```python
from build123d import *

# Parameters (mm, degrees)
SKETCH1_W               = 14
SKETCH1_H               = 15
BOSS_EXTRUDE1_DEPTH     = 4
SKETCH2_R               = 3
SKETCH2_R_2             = 1.5
CUT_EXTRUDE1_DEPTH      = 1
CUT_EXTRUDE1_DEPTH_BACK = 5
FILLET1_R               = 2
CUT_EXTRUDE2_START      = -0.2
SKETCH3_W               = 4
SKETCH3_H               = 6
CUT_EXTRUDE2_DEPTH      = 1.2
LPATTERN1_COUNT         = 4
LPATTERN1_PITCH         = 6.666666667
MIRROR1_START           = -0.2
MIRROR1_COPY_1_SKETCH_W = 4
MIRROR1_COPY_1_SKETCH_H = 6
MIRROR1_COPY_1_DEPTH    = 1.2
MIRROR1_COPY_2_SKETCH_W = 4
MIRROR1_COPY_2_SKETCH_H = 6
MIRROR1_COPY_2_DEPTH    = 1.2
MIRROR1_COPY_3_SKETCH_W = 4
MIRROR1_COPY_3_SKETCH_H = 6
MIRROR1_COPY_3_DEPTH    = 1.2
SKETCH4_W               = 6
SKETCH4_H               = 4
CUT_EXTRUDE3_DEPTH      = 1
CUT_EXTRUDE3_DEPTH_BACK = 0.2


with BuildPart() as part:
    # Sketch1 → Boss-Extrude1 (new body)
    with BuildSketch(Plane(origin=(0, 0, 0), x_dir=(1, 0, 0), z_dir=(0, 1, 0))):
        Polygon((-11, 18), (-11, 7.5), (-11, -7.5), (-11, -18), (25, -18), (25, 18), align=None)
        with Locations((-18, 0)):
            Rectangle(SKETCH1_W, SKETCH1_H)
    extrude(amount=BOSS_EXTRUDE1_DEPTH)

    # Sketch2 → Cut-Extrude1 (cut, two sides)
    with BuildSketch(Plane(origin=(0, 4, 0), x_dir=(1, 0, 0), z_dir=(0, 1, 0))) as cut_extrude1_sk:
        with Locations((-18, 3.75)):
            Circle(SKETCH2_R)
        with Locations((-8.25, 15.25)):
            Circle(SKETCH2_R_2)
        with Locations((22.25, 15.25)):
            Circle(SKETCH2_R_2)
        with Locations((-18, -3.75)):
            Circle(SKETCH2_R)
        with Locations((22.25, -15.25)):
            Circle(SKETCH2_R_2)
        with Locations((-8.25, -15.25)):
            Circle(SKETCH2_R_2)
    extrude(amount=CUT_EXTRUDE1_DEPTH, mode=Mode.SUBTRACT)
    extrude(cut_extrude1_sk.sketch, amount=-CUT_EXTRUDE1_DEPTH_BACK, mode=Mode.SUBTRACT)

    # Fillet1
    fillet1_edges = [part.edges().sort_by_distance(p)[0] for p in [
        (-11, 2, -18),
        (25, 2, -18),
        (25, 2, 18),
        (-11, 2, 18),
        (-11, 2, 7.5),
        (-25, 2, 7.5),
        (-25, 2, -7.5),
        (-11, 2, -7.5),
    ]]
    fillet(fillet1_edges, radius=FILLET1_R)

    # Sketch3 → Cut-Extrude2 (cut)
    with BuildSketch(Plane(origin=(0, 4, 0), x_dir=(1, 0, 0), z_dir=(0, 1, 0)).offset(CUT_EXTRUDE2_START)):
        with Locations((-3.25, 14)):
            Rectangle(SKETCH3_W, SKETCH3_H)
    cut_extrude2 = extrude(amount=CUT_EXTRUDE2_DEPTH, mode=Mode.SUBTRACT)

    # LPattern1: Cut-Extrude2 ×4
    with Locations(*[(i * LPATTERN1_PITCH, 0, 0) for i in range(1, LPATTERN1_COUNT)]):
        add(cut_extrude2, mode=Mode.SUBTRACT)

    # Mirror1: Cut-Extrude2 across plane
    add(cut_extrude2.mirror(Plane.XY), mode=Mode.SUBTRACT)

    # Mirror1 copy 1 sketch → Mirror1 copy 1 (cut)
    with BuildSketch(Plane(origin=(6.666666667, 4, 0), x_dir=(1, 0, 0), z_dir=(0, 1, 0)).offset(MIRROR1_START)):
        with Locations((-3.25, -14)):
            Rectangle(MIRROR1_COPY_1_SKETCH_W, MIRROR1_COPY_1_SKETCH_H)
    extrude(amount=MIRROR1_COPY_1_DEPTH, mode=Mode.SUBTRACT)

    # Mirror1 copy 2 sketch → Mirror1 copy 2 (cut)
    with BuildSketch(Plane(origin=(13.333333333, 4, 0), x_dir=(1, 0, 0), z_dir=(0, 1, 0)).offset(MIRROR1_START)):
        with Locations((-3.25, -14)):
            Rectangle(MIRROR1_COPY_2_SKETCH_W, MIRROR1_COPY_2_SKETCH_H)
    extrude(amount=MIRROR1_COPY_2_DEPTH, mode=Mode.SUBTRACT)

    # Mirror1 copy 3 sketch → Mirror1 copy 3 (cut)
    with BuildSketch(Plane(origin=(20, 4, 0), x_dir=(1, 0, 0), z_dir=(0, 1, 0)).offset(MIRROR1_START)):
        with Locations((-3.25, -14)):
            Rectangle(MIRROR1_COPY_3_SKETCH_W, MIRROR1_COPY_3_SKETCH_H)
    extrude(amount=MIRROR1_COPY_3_DEPTH, mode=Mode.SUBTRACT)

    # Sketch4 → Cut-Extrude3 (cut, two sides)
    with BuildSketch(Plane(origin=(0, 4, 0), x_dir=(1, 0, 0), z_dir=(0, 1, 0))) as cut_extrude3_sk:
        with Locations((21, 6.5)):
            Rectangle(SKETCH4_W, SKETCH4_H)
        with Locations((-7, 6.5)):
            Rectangle(SKETCH4_W, SKETCH4_H)
        with Locations((-7, -6.5)):
            Rectangle(SKETCH4_W, SKETCH4_H)
        with Locations((21, -6.5)):
            Rectangle(SKETCH4_W, SKETCH4_H)
    extrude(amount=CUT_EXTRUDE3_DEPTH, mode=Mode.SUBTRACT)
    extrude(cut_extrude3_sk.sketch, amount=-CUT_EXTRUDE3_DEPTH_BACK, mode=Mode.SUBTRACT)


solid = part.part
```
For this review, take the finished solid that the model builds, in its own axes (mm). A direction names the side the tool comes from. Round coordinates to 2 decimals unless told otherwise and drop trailing zeros. Write each loop counter-clockwise with the first axis right and the second up, starting at its lowest first coordinate (ties: lowest second). Pieces come first, ordered by that corner, then holes.
1) Mouldability with a two-part tool opening along X and no side actions: class faces 1 (the face through (-3, 3.8, -14)), 2 (the face through (5, 0, 0)), 3 (the face through (-20.997, 2.028, -3.882)), 4 (the face through (25, 2, 0)) as +X half, -X half, draft (parallel to the pull), parting line (faces both ways), or undercut.
Answer below:
face 1: undercut
face 2: draft
face 3: undercut
face 4: +X half
2) Machinability: for faces 5 (the face through (-11.57, 2.03, -8.1)), 6 (the face through (-11, 2, 13)), 7 (the face through (21, 3.8, 6)), which of the approach directions +Z, -Z, +X, -X, +Y, -Y give a long, thin tool a straight path to every point of the face, cutting with its end or side? Answer none if there is none.
Answer below:
face 5: -Z, -X, +Y, -Y
face 6: +Z, -X, +Y, -Y
face 7: +Y
3) Take a section at D-D on z = 15.25. Give the boundary of the cut face in (x, y), then the cut area to 3 significant figures.
Answer below:
outline: (-11, 0) - (-9.75, 0) - (-9.75, 4) - (-11, 4) - close; (-6.75, 0) - (20.75, 0) - (20.75, 4) - (18.75, 4) - (18.75, 3.8) - (14.75, 3.8) - (14.75, 4) - (12.08, 4) - (12.08, 3.8) - (8.08, 3.8) - (8.08, 4) - (5.42, 4) - (5.42, 3.8) - (1.42, 3.8) - (1.42, 4) - (-1.25, 4) - (-1.25, 3.8) - (-5.25, 3.8) - (-5.25, 4) - (-6.75, 4) - close; (23.75, 0) - (25, 0) - (25, 4) - (23.75, 4) - close
area: 117 mm2
4) Take a section at C-C on x = 3.5. Give the boundary of the cut face in (y, z).
Answer below:
outline: (0, -18) - (4, -18) - (4, -17) - (3.8, -17) - (3.8, -11) - (4, -11) - (4, 11) - (3.8, 11) - (3.8, 17) - (4, 17) - (4, 18) - (0, 18) - close
5) Take a section at B-B on z = -3.75. Give the boundary of the cut face in (x, y).
Answer below:
outline: (-25, 0) - (-21, 0) - (-21, 4) - (-25, 4) - close; (-15, 0) - (25, 0) - (25, 4) - (-15, 4) - close
6) For line 1 along Z through (x, y) = (-8.25, 2.95); line 2 along X through (y, z) = (1.4, -15.25); line 3 along Z through (x, y) = (-18, 1.2), list the stretches that pass through material, from the lowest coordinate up.
Answer below:
line 1: z = -18 to -16.75, -13.75 to 13.75, 16.75 to 18
line 2: x = -11 to -9.75, -6.75 to 20.75, 23.75 to 25
line 3: z = -7.5 to -6.75, -0.75 to 0.75, 6.75 to 7.5
7) Take a section at A-A on x = -8.25. Give the boundary of the cut face in (y, z).
Answer below:
outline: (0, -18) - (4, -18) - (4, -16.75) - (0, -16.75) - close; (0, -13.75) - (4, -13.75) - (4, -8.5) - (3.8, -8.5) - (3.8, -4.5) - (4, -4.5) - (4, 4.5) - (3.8, 4.5) - (3.8, 8.5) - (4, 8.5) - (4, 13.75) - (0, 13.75) - close; (0, 16.75) - (4, 16.75) - (4, 18) - (0, 18) - close
